The model under review builds one solid part; all positions refer to its coordinate system, in mm. A direction names the side the tool comes from. Round coordinates to 2 decimals unless told otherwise and drop trailing zeros. Write each loop counter-clockwise with the first axis right and the second up, starting at its lowest first coordinate (ties: lowest second). Pieces come first, ordered by that corner, then holes. Notation, with made-up numbers: M 62.25,36.25 L 69.25,36.25 A32 cw 69.25,66.25 Z; hole C 17,33 d4. An arc over 180 degrees is marked long. Write item = value, one per line. Start each with the question number.
Item 1: Take a section at D-D, the plane y = 0. Give the boundary of the cut face in (x, z).
Item 2: For pin 1 Ø12 at (x, y) = (7.5, 3.5) entering from -Z; pin 2 Ø5 at (x, y) = (1, -2) entering from +Z; pin 3 Ø4 at (x, z) = (5, -8) entering from +Y; pin 4 Ø20 at (y, z) = (0, -0.5) entering from -X, all flat-tipped, find the tip position at first contact; note any pin that passes through.
Item 3: The part is to be moulded in two halves that separate along X. For faces 3 (the cylindrical face through (-0.25, -4.88, 1.08)), 4 (the flat face through (15, 9, -9)), 5 (the flat face through (-17.5, -4, -4)), say which applies: +X half, -X half, draft (parallel to the pull), parting line (faces both ways), or undercut.
Item 4: Tool access review of faces 1 (the flat face through (-15, 9, -9)), 2 (the cylindrical face through (-16.233, -19.524, 4.336)): name each direction out of +Z, -Z, +X, -X, +Y, -Y from which nothing blocks a thin tool from reaching the whole face with its end or side.
Item 5: To check wall thickness, follow line 1 along X through (y, z) = (-18, -4); line 2 along Y through (x, z) = (-3, 0); line 3 along Z through (x, y) = (-1, 0.5). State the ranges of each line that lie inside material, in increasing order.
Item 6: Take a section at A-A, the plane z = -16. Give the boundary of the cut face in (x, y).
Item 7: Take a section at C-C, the plane x = 9. Give the boundary of the cut face in (y, z), plus the area to 3 significant figures.
from build123d import *

# Parameters (mm, degrees)
SKETCH1_R               = 12.5
SKETCH1_R_2             = 5
BOSS_EXTRUDE1_DEPTH     = 15
SKETCH2_R               = 20
BOSS_EXTRUDE2_DEPTH     = 2.5
CUT_EXTRUDE1_DEPTH      = 46
CUT_EXTRUDE1_DEPTH_BACK = 46
SKETCH3_R               = 5


with BuildPart() as part:
    # Sketch1 → Boss-Extrude1 (new, symmetric)
    with BuildSketch(Plane(origin=(0, 0, 0), x_dir=(0, 0, -1), z_dir=(1, 0, 0))):
        Circle(SKETCH1_R)
        Circle(SKETCH1_R_2, mode=Mode.SUBTRACT)
    extrude(amount=BOSS_EXTRUDE1_DEPTH, both=True)

    # Sketch2 → Boss-Extrude2 (add)
    with BuildSketch(Plane(origin=(15, 0, 0), x_dir=(0, 0, -1), z_dir=(1, 0, 0))):
        Circle(SKETCH2_R)
    boss_extrude2 = extrude(amount=BOSS_EXTRUDE2_DEPTH)

    # Mirror1: Boss-Extrude2 across plane
    add(boss_extrude2.mirror(Plane(origin=(0, 0, 0), x_dir=(0, 0, 1), z_dir=(1, 0, 0))))

    # Sketch3 → Cut-Extrude1 (cut, two sides: drawn at the far end of the back side and taken through both)
    with BuildSketch(Plane(origin=(17.5, 0, 0), x_dir=(0, 0, -1), z_dir=(1, 0, 0)).offset(-CUT_EXTRUDE1_DEPTH_BACK)):
        Circle(SKETCH3_R)
    extrude(amount=CUT_EXTRUDE1_DEPTH + CUT_EXTRUDE1_DEPTH_BACK, mode=Mode.SUBTRACT)


solid = part.part
Response values:
q1.outline = M -17.5,-20 L -15,-20 L -15,-12.5 L 15,-12.5 L 15,-20 L 17.5,-20 L 17.5,-5 L -17.5,-5 Z; M -17.5,5 L 17.5,5 L 17.5,20 L 15,20 L 15,12.5 L -15,12.5 L -15,20 L -17.5,20 Z
q2.pin_1 = -12.5
q2.pin_2 = 12.5
q2.pin_3 = 10.97
q2.pin_4 = -17.5
q3.face_3 = draft
q3.face_4 = undercut
q3.face_5 = -X half
q4.face_1 = none
q4.face_2 = +X, -X
q5.line_1 = -17.5 to -15, 15 to 17.5
q5.line_2 = -12.5 to -5, 5 to 12.5
q5.line_3 = -12.49 to -4.97, 4.97 to 12.49
q6.outline = M -17.5,-12 L -15,-12 L -15,12 L -17.5,12 Z; M 15,-12 L 17.5,-12 L 17.5,12 L 15,12 Z
q7.outline = C 0,0 d25; hole C 0,0 d10
q7.area = 412 mm2
